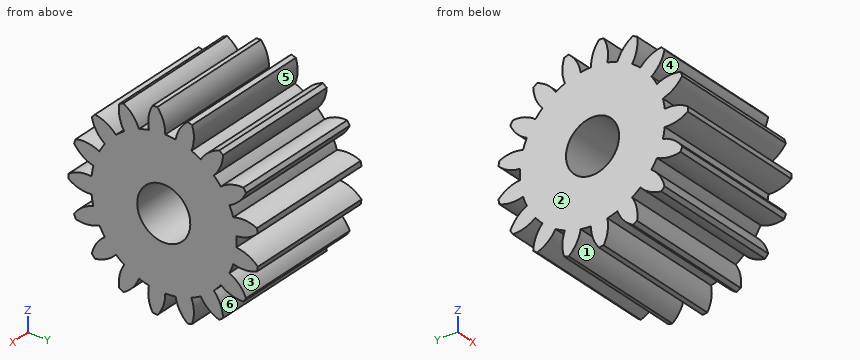
from build123d import *

# Parameters (mm, degrees)
SPUR_START             = -92.950977625
SPUR_GEAR_AM_OUTLINE_R = 1.5
SPUR_GEAR_AM_DEPTH     = 8.001
SKETCH1_R              = 1.5875
CUT_EXTRUDE1_DEPTH     = 50.509189617


# Read off the part's stored shape, not the designer's step: spur gear_am
with BuildPart() as part:
    # spur gear_am outline → spur gear_am (new body)
    with BuildSketch(Plane.YZ.offset(SPUR_START)):
        with BuildLine():
            ThreePointArc((31.652652911, 27.663945588), (31.729301927, 27.784343625), (31.802912423, 27.906623033))
            ThreePointArc((31.802912423, 27.906623033), (31.401254023, 28.50628356), (30.815920965, 28.928548203))
            ThreePointArc((30.815920965, 28.928548203), (30.938385979, 29.213966947), (31.040168606, 29.50739809))
            ThreePointArc((31.040168606, 29.50739809), (31.757212806, 29.425119095), (32.45803063, 29.597678058))
            ThreePointArc((32.45803063, 29.597678058), (32.486010922, 29.737634702), (32.510478248, 29.878248033))
            ThreePointArc((32.510478248, 29.878248033), (31.919320576, 30.292319071), (31.220974171, 30.474622435))
            ThreePointArc((31.220974171, 30.474622435), (31.232064254, 30.785006953), (31.220974171, 31.095391471))
            ThreePointArc((31.220974171, 31.095391471), (31.919320576, 31.277694835), (32.510478248, 31.691765874))
            ThreePointArc((32.510478248, 31.691765874), (32.486010922, 31.832379205), (32.45803063, 31.972335848))
            ThreePointArc((32.45803063, 31.972335848), (31.757212806, 32.144894811), (31.040168606, 32.062615816))
            ThreePointArc((31.040168606, 32.062615816), (30.938385979, 32.356046959), (30.815920965, 32.641465703))
            ThreePointArc((30.815920965, 32.641465703), (31.401254023, 33.063730346), (31.802912423, 33.663390873))
            ThreePointArc((31.802912423, 33.663390873), (31.729301927, 33.785670282), (31.652652911, 33.906068318))
            ThreePointArc((31.652652911, 33.906068318), (30.936824265, 33.81381016), (30.297923062, 33.47806104))
            ThreePointArc((30.297923062, 33.47806104), (30.097014035, 33.714909307), (29.879713667, 33.936814893))
            ThreePointArc((29.879713667, 33.936814893), (30.272980906, 34.542011636), (30.430893842, 35.246274174))
            ThreePointArc((30.430893842, 35.246274174), (30.318081681, 35.333705149), (30.203115814, 35.418284156))
            ThreePointArc((30.203115814, 35.418284156), (29.568952972, 35.073668852), (29.094481914, 34.529794388))
            ThreePointArc((29.094481914, 34.529794388), (28.821580363, 34.678072107), (28.538792261, 34.806494957))
            ThreePointArc((28.538792261, 34.806494957), (28.68688076, 35.512888625), (28.579721215, 36.226638616))
            ThreePointArc((28.579721215, 36.226638616), (28.442943297, 36.267413119), (28.305187358, 36.304750233))
            ThreePointArc((28.305187358, 36.304750233), (27.838337524, 35.754319991), (27.592376558, 35.075773441))
            ThreePointArc((27.592376558, 35.075773441), (27.284339349, 35.115454886), (26.974255613, 35.133050782))
            ThreePointArc((26.974255613, 35.133050782), (26.8571652, 35.845238996), (26.499405664, 36.472080549))
            ThreePointArc((26.499405664, 36.472080549), (26.357134605, 36.460691758), (26.215193296, 36.445744395))
            ThreePointArc((26.215193296, 36.445744395), (25.978707128, 35.763837869), (25.994474644, 35.042260705))
            ThreePointArc((25.994474644, 35.042260705), (25.69290391, 34.967986675), (25.397403066, 34.872379194))
            ThreePointArc((25.397403066, 34.872379194), (25.030947451, 35.494176991), (24.470905332, 35.94945168))
            ThreePointArc((24.470905332, 35.94945168), (24.342355626, 35.887437714), (24.215398907, 35.822224598))
            ThreePointArc((24.215398907, 35.822224598), (24.241215173, 35.100937042), (24.51658168, 34.433782259))
            ThreePointArc((24.51658168, 34.433782259), (24.26220622, 34.255583875), (24.021197296, 34.059685336))
            ThreePointArc((24.021197296, 34.059685336), (23.454868339, 34.507115477), (22.768180428, 34.729335933))
            ThreePointArc((22.768180428, 34.729335933), (22.670713426, 34.625072122), (22.575887506, 34.518400646))
            ThreePointArc((22.575887506, 34.518400646), (22.860519576, 33.855145941), (23.358295302, 33.332516489))
            ThreePointArc((23.358295302, 33.332516489), (23.18546993, 33.074460429), (23.031502516, 32.804728017))
            ThreePointArc((23.031502516, 32.804728017), (22.341786081, 33.017362582), (21.621193386, 32.976516701))
            ThreePointArc((21.621193386, 32.976516701), (21.567972546, 32.84408445), (21.518084191, 32.710361188))
            ThreePointArc((21.518084191, 32.710361188), (22.023090926, 32.194715558), (22.676048502, 31.88719544))
            ThreePointArc((22.676048502, 31.88719544), (22.608114243, 31.584133606), (22.561982491, 31.276996177))
            ThreePointArc((22.561982491, 31.276996177), (21.842028605, 31.22611769), (21.184851162, 30.927721934))
            ThreePointArc((21.184851162, 30.927721934), (21.183064254, 30.785006953), (21.184851162, 30.642291972))
            ThreePointArc((21.184851162, 30.642291972), (21.842028605, 30.343896216), (22.561982491, 30.293017729))
            ThreePointArc((22.561982491, 30.293017729), (22.608114243, 29.9858803), (22.676048502, 29.682818466))
            ThreePointArc((22.676048502, 29.682818466), (22.023090926, 29.375298348), (21.518084191, 28.859652718))
            ThreePointArc((21.518084191, 28.859652718), (21.567972546, 28.725929456), (21.621193386, 28.593497205))
            ThreePointArc((21.621193386, 28.593497205), (22.341786081, 28.552651324), (23.031502516, 28.765285889))
            ThreePointArc((23.031502516, 28.765285889), (23.18546993, 28.495553477), (23.358295302, 28.237497417))
            ThreePointArc((23.358295302, 28.237497417), (22.860519576, 27.714867965), (22.575887506, 27.051613261))
            ThreePointArc((22.575887506, 27.051613261), (22.670713426, 26.944941784), (22.768180428, 26.840677973))
            ThreePointArc((22.768180428, 26.840677973), (23.454868339, 27.062898429), (24.021197296, 27.51032857))
            ThreePointArc((24.021197296, 27.51032857), (24.26220622, 27.314430032), (24.51658168, 27.136231648))
            ThreePointArc((24.51658168, 27.136231648), (24.241215173, 26.469076865), (24.215398907, 25.747789309))
            ThreePointArc((24.215398907, 25.747789309), (24.342355626, 25.682576192), (24.470905332, 25.620562226))
            ThreePointArc((24.470905332, 25.620562226), (25.030947451, 26.075836915), (25.397403066, 26.697634712))
            ThreePointArc((25.397403066, 26.697634712), (25.69290391, 26.602027231), (25.994474644, 26.527753202))
            ThreePointArc((25.994474644, 26.527753202), (25.978707128, 25.806176038), (26.215193296, 25.124269511))
            ThreePointArc((26.215193296, 25.124269511), (26.357134605, 25.109322148), (26.499405664, 25.097933357))
            ThreePointArc((26.499405664, 25.097933357), (26.8571652, 25.72477491), (26.974255613, 26.436963124))
            ThreePointArc((26.974255613, 26.436963124), (27.284339349, 26.45455902), (27.592376558, 26.494240465))
            ThreePointArc((27.592376558, 26.494240465), (27.838337524, 25.815693915), (28.305187358, 25.265263673))
            ThreePointArc((28.305187358, 25.265263673), (28.442943297, 25.302600787), (28.579721215, 25.34337529))
            ThreePointArc((28.579721215, 25.34337529), (28.68688076, 26.057125281), (28.538792261, 26.763518949))
            ThreePointArc((28.538792261, 26.763518949), (28.821580363, 26.891941799), (29.094481914, 27.040219519))
            ThreePointArc((29.094481914, 27.040219519), (29.568952972, 26.496345054), (30.203115814, 26.151729751))
            ThreePointArc((30.203115814, 26.151729751), (30.318081681, 26.236308758), (30.430893842, 26.323739732))
            ThreePointArc((30.430893842, 26.323739732), (30.272980906, 27.02800227), (29.879713667, 27.633199013))
            ThreePointArc((29.879713667, 27.633199013), (30.097014035, 27.855104599), (30.297923062, 28.091952866))
            ThreePointArc((30.297923062, 28.091952866), (30.936824265, 27.756203746), (31.652652911, 27.663945588))
        make_face()
        with Locations((26.883064254, 30.785006953)):
            Circle(SPUR_GEAR_AM_OUTLINE_R, mode=Mode.SUBTRACT)
    extrude(amount=SPUR_GEAR_AM_DEPTH)

    # Sketch1 → Cut-Extrude1 (cut, through all)
    with BuildSketch(Plane(origin=(-84.949977625, 0, 0), x_dir=(0, 0, -1), z_dir=(1, 0, 0))):
        with Locations((-30.785006953, 26.883064254)):
            Circle(SKETCH1_R)
    extrude(amount=-CUT_EXTRUDE1_DEPTH, mode=Mode.SUBTRACT)


solid = part.part
Verification items for the finished model (mm, model axes). Face numbers are marked on the shaded views. A direction names the side the tool comes from. Coordinates: 2 decimals unless noted, no trailing zeros. Order: outer loops, then holes, each group sorted by start corner. A loop starts at its lowest first (then second) coordinate and runs counter-clockwise, first axis right, second up.
1. Sectioned sample at A-A, the plane y = 25.75. Record the cut outline in (x, z).
Results found:
outline: (-92.95, 26.59) - (-84.95, 26.59) - (-84.95, 29.67) - (-92.95, 29.67) - close; (-92.95, 31.9) - (-84.95, 31.9) - (-84.95, 34.98) - (-92.95, 34.98) - close
2. Scan lines: line 1 (Z direction, x = -89.75, y = 23); line 2 (Z direction, x = -90.75, y = 22.5); line 3 (Z direction, x = -90.5, y = 28). Record each from-to range of solid material in increasing order.
Results found:
line 1: z = 26.89 to 27.9, 28.75 to 32.82, 33.67 to 34.68
line 2: z = 28.58 to 29.63, 30.29 to 31.28, 31.94 to 32.99
line 3: z = 25.58 to 29.66, 31.91 to 35.99
3. Go/stop test with a flat-tipped pin: pin 1 Ø1 at (x, y) = (-88, 28.5) entering from +Z. Record where the tip stops, or that it passes through.
Results found:
pin 1: stops at z = 36.3
4. Release check for a two-part mould opening along Z. For the marked faces 1, 2 and 3 record: +Z half, -Z half, draft (parallel to the pull), parting line (faces both ways), or undercut.
Results found:
face 1: -Z half
face 2: draft
face 3: undercut
5. Sectioned sample at B-B, the plane z = 26. Record the cut outline in (x, y), and give its area (3 significant figures).
Results found:
outline: (-92.95, 24.2) - (-84.95, 24.2) - (-84.95, 24.96) - (-92.95, 24.96) - close; (-92.95, 25.96) - (-84.95, 25.96) - (-84.95, 26.93) - (-92.95, 26.93) - close; (-92.95, 27.74) - (-84.95, 27.74) - (-84.95, 28.69) - (-92.95, 28.69) - close
area: 21.5 mm2
6. Set-up check for the marked faces 4, 5 and 6: record each of +Z, -Z, +X, -X, +Y, -Y from which the full face is reachable in a straight line by a thin tool's end or side.
Results found:
face 4: +X, -X, -Y
face 5: +X, -X
face 6: +X, -X, +Y
